Input: part model. Units: mm. Frame: model coordinates. Give positions to 0.01 mm unless a question says otherwise; leave off trailing zeros. Write each loop counter-clockwise with the first axis right and the second up, starting at its lowest first coordinate (ties: lowest second). Pieces come first, ordered by that corner, then holes.
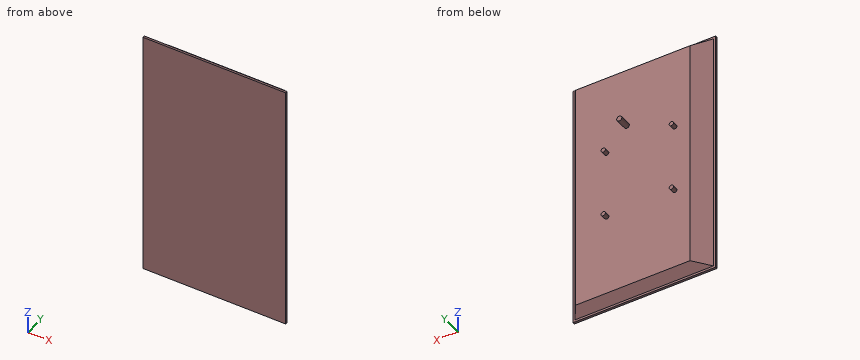
```python
from build123d import *

# Parameters (mm, degrees)
F0_W      = 419.1
F0_H      = 726.44
F1_DEPTH  = 6.35
F4_DEPTH  = 44.45
F5_R      = 7.62
F6_DEPTH  = 63.5
F8_W      = 336.55
F8_H      = 675.64
F9_W      = 406.4
F9_H      = 713.74
F11_DEPTH = 28.575


with BuildPart() as f1:
    # F0 (on Front) → F1 (new body)
    with BuildSketch(Plane.XZ):
        Rectangle(F0_W, F0_H)
    extrude(amount=-F1_DEPTH)

    # F2 (on face) → F4 (join)
    with BuildSketch(Plane(origin=(0, 6.35, 0), x_dir=(-1, 0, 0), z_dir=(0, 1, 0))):
        with BuildLine():
            ThreePointArc((113.9, 101.22), (107.55, 107.57), (101.2, 101.22))
            Line((101.2, 101.22), (107.55, 101.22))
            Line((107.55, 101.22), (107.55, 94.87))
            ThreePointArc((107.55, 94.87), (112.0401280605, 96.7298719395), (113.9, 101.22))
        make_face()
        with BuildLine():
            Line((107.55, 101.22), (101.2, 101.22))
            ThreePointArc((101.2, 101.22), (103.0598719395, 96.7298719395), (107.55, 94.87))
            Line((107.55, 94.87), (107.55, 101.22))
        make_face()
        with BuildLine():
            Line((-92.45, 101.22), (-86.1, 101.22))
            ThreePointArc((-86.1, 101.22), (-96.9401280605, 105.7101280605), (-92.45, 94.87))
            Line((-92.45, 94.87), (-92.45, 101.22))
        make_face()
        with BuildLine():
            ThreePointArc((-92.45, 94.87), (-87.9598719395, 96.7298719395), (-86.1, 101.22))
            Line((-86.1, 101.22), (-92.45, 101.22))
            Line((-92.45, 101.22), (-92.45, 94.87))
        make_face()
        with BuildLine():
            Line((107.55, -98.78), (107.55, -92.43))
            ThreePointArc((107.55, -92.43), (103.0598719395, -94.2898719395), (101.2, -98.78))
            Line((101.2, -98.78), (107.55, -98.78))
        make_face()
        with BuildLine():
            ThreePointArc((113.9, -98.78), (112.0401280605, -94.2898719395), (107.55, -92.43))
            Line((107.55, -92.43), (107.55, -98.78))
            Line((107.55, -98.78), (101.2, -98.78))
            ThreePointArc((101.2, -98.78), (107.55, -105.13), (113.9, -98.78))
        make_face()
        with BuildLine():
            ThreePointArc((-86.1, -98.78), (-87.9598719395, -94.2898719395), (-92.45, -92.43))
            Line((-92.45, -92.43), (-92.45, -98.78))
            Line((-92.45, -98.78), (-86.1, -98.78))
        make_face()
        with BuildLine():
            Line((-92.45, -98.78), (-92.45, -92.43))
            ThreePointArc((-92.45, -92.43), (-96.9401280605, -103.2701280605), (-86.1, -98.78))
            Line((-86.1, -98.78), (-92.45, -98.78))
        make_face()
    extrude(amount=F4_DEPTH)

    # F5 (on face) → F6 (join)
    with BuildSketch(Plane(origin=(0, 6.35, 0), x_dir=(-1, 0, 0), z_dir=(0, 1, 0))):
        with Locations((-33.45, 163.22)):
            Circle(F5_R)
    extrude(amount=F6_DEPTH)

    # F8 (on offset) → F10 section 0
    with BuildSketch(Plane(origin=(0, 34.925, 0), x_dir=(-1, 0, 0), z_dir=(0, 1, 0))):
        with Locations((-15.875, 0)):
            Rectangle(F8_W, F8_H)
    # F9 (on face) → F10 section 1
    with BuildSketch(Plane(origin=(0, 6.35, 0), x_dir=(-1, 0, 0), z_dir=(0, 1, 0))):
        Rectangle(F9_W, F9_H)
    loft()

    # F8 (on offset) → F11 (join)
    with BuildSketch(Plane(origin=(0, 34.925, 0), x_dir=(-1, 0, 0), z_dir=(0, 1, 0))):
        with Locations((-15.875, 0)):
            Rectangle(F8_W, F8_H)
    extrude(amount=-F11_DEPTH)


solid = f1.part
```
Item 1: Section A-A (y = 62.5). Return loops of the section in (x, z), and give its area (3 significant figures).
Item 2: Pin query (flat end, axial travel): pin 1 (10 mm diameter, centred on x = -107, z = -96, fed in from +Y); pin 2 (1.5 mm diameter, centred on x = -142, y = 34.5, fed in from -Z); pin 3 (6 mm diameter, centred on x = 148, z = -76.5, fed in from +Y) (3 decimals). Return the tip coordinate at first contact, or that it passes through.
Item 3: Ray query, line 1 (Y direction, x = 26, z = 198) (3 decimals); line 2 (Z direction, x = -133, y = 14); line 3 (Z direction, x = -84, y = 34). Return the intervals inside material, ascending.
Solved:
1. outline: circle Ø15.24 at (33.45, 163.22)
1. area: 182 mm2
2. pin 1: stops at y = 50.8
2. pin 2: stops at z = -338.6
2. pin 3: stops at y = 34.925
3. line 1: y = 0 to 34.925
3. line 2: z = -351.77 to 351.77
3. line 3: z = -338.44 to 338.44
